```python
from build123d import *

# Parameters (mm, degrees)
SKETCH1_W           = 8
SKETCH1_H           = 4
SKETCH1_R           = 3
BOSS_EXTRUDE1_DEPTH = 37
SKETCH3_W           = 8
SKETCH3_H           = 4
BOSS_EXTRUDE2_DEPTH = 13
SKETCH4_W           = 20
SKETCH4_H           = 4
BOSS_EXTRUDE3_DEPTH = 30
FILLET1_R           = 10
SKETCH5_W           = 9
SKETCH5_H           = 10
SKETCH5_H_2         = 17
CUT_EXTRUDE1_DEPTH  = 19


with BuildPart() as part:
    # Sketch1 → Boss-Extrude1 (new body)
    # profile 1 of 2: a face of its own
    with BuildSketch(Plane.XY):
        with Locations((37.629567615, 21.902115813)):
            Rectangle(SKETCH1_W, SKETCH1_H)
    # profile 2 of 2: a face of its own
    with BuildSketch(Plane.XY):
        with BuildLine():
            ThreePointArc((41.629567615, 32.902115813), (46.129567615, 37.402115813), (50.629567615, 32.902115813))
            Line((50.629567615, 32.902115813), (50.629567615, 19.902115813))
            Line((50.629567615, 19.902115813), (41.629567615, 19.902115813))
            Line((41.629567615, 19.902115813), (41.629567615, 23.902115813))
            Line((41.629567615, 23.902115813), (41.629567615, 32.902115813))
        make_face()
        with Locations((46.129567615, 32.902115813)):
            Circle(SKETCH1_R, mode=Mode.SUBTRACT)
    extrude(amount=BOSS_EXTRUDE1_DEPTH)

    # Sketch3 → Boss-Extrude2 (add)
    with BuildSketch(Plane(origin=(0, 0, 0), x_dir=(-1, 0, 0), z_dir=(0, 0, -1))):
        with Locations((-37.629567615, 21.902115813)):
            Rectangle(SKETCH3_W, SKETCH3_H)
    extrude(amount=BOSS_EXTRUDE2_DEPTH)

    # Sketch4 → Boss-Extrude3 (add)
    with BuildSketch(Plane(origin=(0, 0, -13), x_dir=(-1, 0, 0), z_dir=(0, 0, -1))):
        with Locations((-31.629567615, 21.902115813)):
            Rectangle(SKETCH4_W, SKETCH4_H)
    extrude(amount=BOSS_EXTRUDE3_DEPTH)

    # Fillet1
    # the kernel refuses this fillet: 10 mm, written as the material it takes off along each edge
    with BuildSketch(Plane(origin=(21.629567615, 19.902115813, 7), x_dir=(1, 0, 0), z_dir=(0, 0, -1))) as fillet1_piece_1:
        with BuildLine():
            CenterArc((8, -10), FILLET1_R, 90, 53.130102354)
            Line((0, -4), (-0.16, -3.88))
            ThreePointArc((-0.16, -3.88), (-0.2, -2), (-0.2, 0))
            Line((-0.2, 0), (0, 0.2))
            Line((0, 0.2), (8, 0.2))
            Line((8, 0.2), (8, 0))
        make_face()
    extrude(amount=70, mode=Mode.SUBTRACT)

    # Sketch5 → Cut-Extrude1 (cut)
    with BuildSketch(Plane(origin=(0, 19.902115813, 0), x_dir=(-1, 0, 0), z_dir=(0, -1, 0))):
        with Locations((-46.129567615, -5)):
            Rectangle(SKETCH5_W, SKETCH5_H)
        with Locations((-46.129567615, -23.5)):
            Rectangle(SKETCH5_W, SKETCH5_H_2)
    extrude(amount=-CUT_EXTRUDE1_DEPTH, mode=Mode.SUBTRACT)


solid = part.part
```
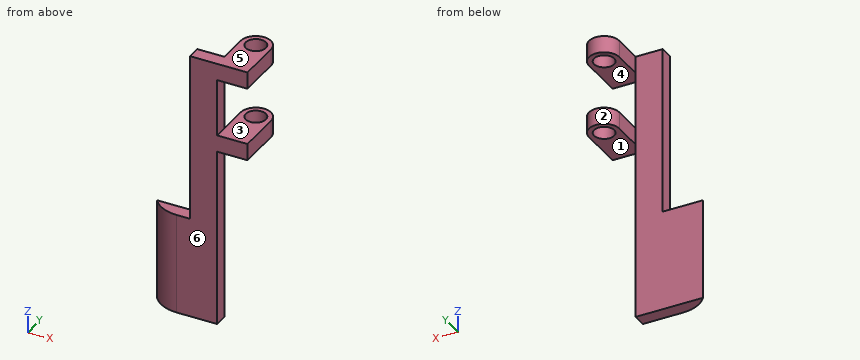
CAD build for the part. Positions are in the model's coordinates, mm. Face numbers are marked on the shaded views. A direction names the side the tool comes from. Round coordinates to 2 decimals unless told otherwise and drop trailing zeros. Order: outer loops, then holes, each group sorted by start corner. A loop starts at its lowest first (then second) coordinate and runs counter-clockwise, first axis right, second up. Notation, with made-up numbers: (-22.5, 67.25) -> (16.5, 67.25) arc R16 cw to (16.5, 75.25) -> close; hole circle Ø8 at (56, 5). An arc over 180 degrees is marked (long way). One line per question, with ' | ' between items.
Q1. Probe probe 1 along Z at (x, y) = (47.5, 25); probe 2 along Y at (x, z) = (38.75, -33); probe 3 along X at (y, z) = (23.75, 25). List the from-to ranges inside material, lowest first.
Completed:
probe 1: z = 10 to 15, 32 to 37 | probe 2: y = 19.9 to 23.9 | probe 3: x = 33.63 to 41.63
Q2. Two-plate mould, pull along Z, no slides. Class the marked faces 3, 4, 5 and 6: released by +Z, released by -Z, zero draft, split by the parting line, or undercut.
Completed:
face 3: undercut | face 4: undercut | face 5: released by +Z | face 6: zero draft
Q3. Slice it at A-A (y = 27.5). Write the cut outline in (x, z).
Completed:
outline: (41.63, 10) -> (50.63, 10) -> (50.63, 15) -> (41.63, 15) -> close; (41.63, 32) -> (50.63, 32) -> (50.63, 37) -> (41.63, 37) -> close
Q4. Slice it at D-D (x = 31). Write the cut outline in (y, z).
Completed:
outline: (19.9, -43) -> (23.9, -43) -> (23.9, -13) -> (19.9, -13) -> close
Q5. Slice it at B-B (x = 44.5). Write the cut outline in (y, z), then the cut area to 3 significant figures.
Completed:
outline: (19.9, 10) -> (30.38, 10) -> (30.38, 15) -> (19.9, 15) -> close; (19.9, 32) -> (30.38, 32) -> (30.38, 37) -> (19.9, 37) -> close; (35.42, 10) -> (37.1, 10) -> (37.1, 15) -> (35.42, 15) -> close; (35.42, 32) -> (37.1, 32) -> (37.1, 37) -> (35.42, 37) -> close | area: 122 mm^2
Q6. Which spindle directions (+Z, -Z, +X, -X, +Y, -Y) get a long thin tool onto all of the face, cutting with end or side? Do the marked faces 1 and 2. Say none if no direction does.
Completed:
face 1: -Z, +X, +Y, -Y | face 2: +Z, -Z, +Y
Q7. Drop flat-ended pins along their axis: pin 1 (1.5 mm diameter, centred on y = 22, z = 11.5, fed in from -X); pin 2 (4 mm diameter, centred on y = 27.5, z = 33.5, fed in from -X); pin 3 (3 mm diameter, centred on x = 38.5, z = 27.5, fed in from +Y). Give the stop position or say it passes through.
Completed:
pin 1: stops at x = 33.63 | pin 2: stops at x = 41.63 | pin 3: stops at y = 23.9
Q8. Slice it at C-C (y = 31). Write the cut outline in (x, z), then the cut area to 3 significant figures.
Completed:
outline: (41.63, 10) -> (43.81, 10) -> (43.81, 15) -> (41.63, 15) -> close; (41.63, 32) -> (43.81, 32) -> (43.81, 37) -> (41.63, 37) -> close; (48.45, 10) -> (50.63, 10) -> (50.63, 15) -> (48.45, 15) -> close; (48.45, 32) -> (50.63, 32) -> (50.63, 37) -> (48.45, 37) -> close | area: 43.6 mm^2
